```python
from build123d import *

# Parameters (mm, degrees)
SKETCH3_R           = 15.24
BOSS_EXTRUDE2_DEPTH = 10.16
SKETCH4_R           = 6.224057783
BOSS_EXTRUDE3_DEPTH = 5.08
SKETCH5_R           = 12.7
CUT_EXTRUDE1_DEPTH  = 5.08
FILLET1_R           = 6.096
FILLET2_R           = 0.762
FILLET3_R           = 0.254
SKETCH6_W           = 6.35
SKETCH6_H           = 6.35
CUT_EXTRUDE2_DEPTH  = 11


with BuildPart() as part:
    # Sketch1 → Revolve1 (revolve)
    with BuildSketch(Plane(origin=(0, 0, 0), x_dir=(1, 0, 0), z_dir=(0, 1, 0)), mode=Mode.PRIVATE) as revolve1_sk:
        Polygon((0, 5.683021583), (0, -1.936978417), (30.48, -1.936978417), (25.4, 5.683021583), align=None)
    revolve(revolve1_sk.sketch.rotate(Axis((0, 0, -5.683021583), (0, 0, 1)), 180), axis=Axis((0, 0, -5.683021583), (0, 0, 1)))

    # Sketch3 → Boss-Extrude2 (add)
    with BuildSketch(Plane.XY.offset(1.936978417)):
        Circle(SKETCH3_R)
    extrude(amount=BOSS_EXTRUDE2_DEPTH)

    # Sketch4 → Boss-Extrude3 (add)
    with BuildSketch(Plane.XY.offset(12.096978417)):
        Circle(SKETCH4_R)
    extrude(amount=BOSS_EXTRUDE3_DEPTH)

    # Sketch5 → Cut-Extrude1 (cut)
    with BuildSketch(Plane(origin=(0, 0, -5.683021583), x_dir=(-1, 0, 0), z_dir=(0, 0, -1))):
        Circle(SKETCH5_R)
    extrude(amount=-CUT_EXTRUDE1_DEPTH, mode=Mode.SUBTRACT)

    # Fillet1
    fillet1_edges = [part.edges().sort_by_distance(p)[0] for p in [
        (25.4, 0, -5.683021583),
    ]]
    fillet(fillet1_edges, radius=FILLET1_R)

    # Fillet2
    fillet2_edges = [part.edges().sort_by_distance(p)[0] for p in [
        (-15.24, 0, 12.096978417),
        (-6.224057783, 0, 12.096978417),
        (-6.224057783, 0, 17.176978417),
    ]]
    fillet(fillet2_edges, radius=FILLET2_R)

    # Fillet3
    fillet3_edges = [part.edges().sort_by_distance(p)[0] for p in [
        (30.48, 0, 1.936978417),
    ]]
    fillet(fillet3_edges, radius=FILLET3_R)

    # Sketch6 → Cut-Extrude2 (cut)
    with BuildSketch(Plane.XY.offset(17.176978417)):
        Rectangle(SKETCH6_W, SKETCH6_H)
    extrude(amount=-CUT_EXTRUDE2_DEPTH, mode=Mode.SUBTRACT)


solid = part.part
```
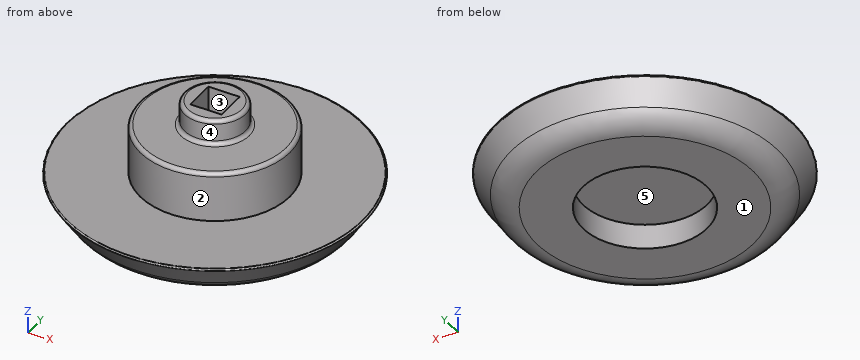
Work out the finished part from the listing and answer in its coordinate system (mm). Face numbers are marked on the shaded views. A direction names the side the tool comes from. Give positions to 0.01 mm unless a question says otherwise; leave off trailing zeros. Order: outer loops, then holes, each group sorted by start corner. A loop starts at its lowest first (then second) coordinate and runs counter-clockwise, first axis right, second up.
1. Section C-C, the plane z = 14 is taken. Determine the outline of the cut face in (x, y) (3 decimals).
Result sheet:
outline: circle Ø12.448 at (0, 0); hole (-3.175, -3.175) - (3.175, -3.175) - (3.175, 3.175) - (-3.175, 3.175) - close
2. Each of these flat-tipped pins is pushed along its axis until it touches: P1, Ø10, axis at x = 22.5, z = 4, coming from the +Y side; P2, Ø3, axis at x = -0.5, y = 1, coming from the +Z side; P3, Ø3, axis at y = -0.5, z = 10, coming from the -X side. Where does it stop, or does it pass through?
Result sheet:
P1: stops at y = 24.29
P2: stops at z = 6.18
P3: stops at x = -15.24
3. For the marked faces 4 and 5, determine the directions among +Z, -Z, +X, -X, +Y, -Y from which every point of the face is accessible in a straight line to the end or side of a thin tool.
Result sheet:
face 4: +Z
face 5: -Z
4. The mould has two halves that part along Y. Classify the marked faces 1, 2 and 3: released by +Y, released by -Y, zero draft, split by the parting line, or undercut.
Result sheet:
face 1: zero draft
face 2: split by the parting line
face 3: undercut
5. Straight lines are drawn through the part: L1, parallel to Z at x = -7, y = 5.5; L2, parallel to Z at x = 19, y = 12; L3, parallel to X at y = 4.5, z = -3.25. For each, find the intervals that lie inside material, in ascending order.
Result sheet:
L1: z = -0.6 to 12.1
L2: z = -5.67 to 1.94
L3: x = -26.63 to -11.88, 11.88 to 26.63
6. Section D-D, the plane z = 10.5 is taken. Determine the outline of the cut face in (x, y) (3 decimals).
Result sheet:
outline: circle Ø30.48 at (0, 0); hole (-3.175, -3.175) - (3.175, -3.175) - (3.175, 3.175) - (-3.175, 3.175) - close
